Read the model definition and answer for the solid it produces. Units are mm, in the model's axes. A direction names the side the tool comes from. Round coordinates to 2 decimals unless told otherwise and drop trailing zeros. Order: outer loops, then holes, each group sorted by start corner. A loop starts at its lowest first (then second) coordinate and runs counter-clockwise, first axis right, second up.
from build123d import *

# Parameters (mm, degrees)
F0_R     = 19.05
F1_DEPTH = 1828.8
F3_START = -25.4
F2_R     = 355.6
F3_DEPTH = 1498.6


with BuildPart() as f1:
    # F0 (on Right) → F1 (new body)
    with BuildSketch(Plane.YZ):
        Circle(F0_R)
    extrude(amount=-F1_DEPTH)

    # F2 (on face) → F3 (join)
    with BuildSketch(Plane(origin=(-1828.8, 0, 0), x_dir=(0, -1, 0), z_dir=(-1, 0, 0)).offset(F3_START)):
        Circle(F2_R)
    extrude(amount=-F3_DEPTH)


solid = f1.part
Q1. A cutting plane is placed at C-C, the plane x = -209.5. Give the vertices of the cut face in (y, z).
Outcome:
outline: circle Ø38.1 at (0, 0)
Q2. Straight lines are drawn through the part: probe 1 along X at (y, z) = (169, 30.5); probe 2 along Z at (x, y) = (-1341, -7); probe 3 along Z at (x, y) = (-503, 13). For each, find the intervals that lie inside material, in ascending order.
Outcome:
probe 1: x = -1803.4 to -304.8
probe 2: z = -355.53 to 355.53
probe 3: z = -355.36 to 355.36
Q3. A cutting plane is placed at D-D, the plane x = -822. Give the vertices of the cut face in (y, z), plus the area to 3 significant figures.
Outcome:
outline: circle Ø711.2 at (0, 0)
area: 397,000 mm2
Q4. For faces 1 (the face through (-1064.59, -339.18, 106.81)), 2 (the face through (-1815.92, -15.12, -11.59)), 3 (the face through (-150.27, -15.12, -11.59)), determine the directions among +Z, -Z, +X, -X, +Y, -Y from which every point of the face is accessible in a straight line to the end or side of a thin tool.
Outcome:
face 1: +X, -X
face 2: -X
face 3: +X
Q5. Flat-ended cylindrical pins translate along their axes: pin 1 (6 mm diameter, centred on x = -397, z = -231, fed in from -Y); pin 2 (8 mm diameter, centred on x = -1393.5, y = 153, fed in from +Z); pin 3 (1 mm diameter, centred on x = -438.5, y = 138, fed in from -Z). Find the tip coordinate at first contact, or state that the pin passes through.
Outcome:
pin 1: stops at y = -272.89
pin 2: stops at z = 322.88
pin 3: stops at z = -327.94
Q6. A cutting plane is placed at A-A, the plane z = 0. Give the vertices of the cut face in (x, y), plus the area to 3 significant figures.
Outcome:
outline: (-1828.8, -19.05) - (-1803.4, -19.05) - (-1803.4, -355.6) - (-304.8, -355.6) - (-304.8, -19.05) - (0, -19.05) - (0, 19.05) - (-304.8, 19.05) - (-304.8, 355.6) - (-1803.4, 355.6) - (-1803.4, 19.05) - (-1828.8, 19.05) - close
area: 1,080,000 mm2
